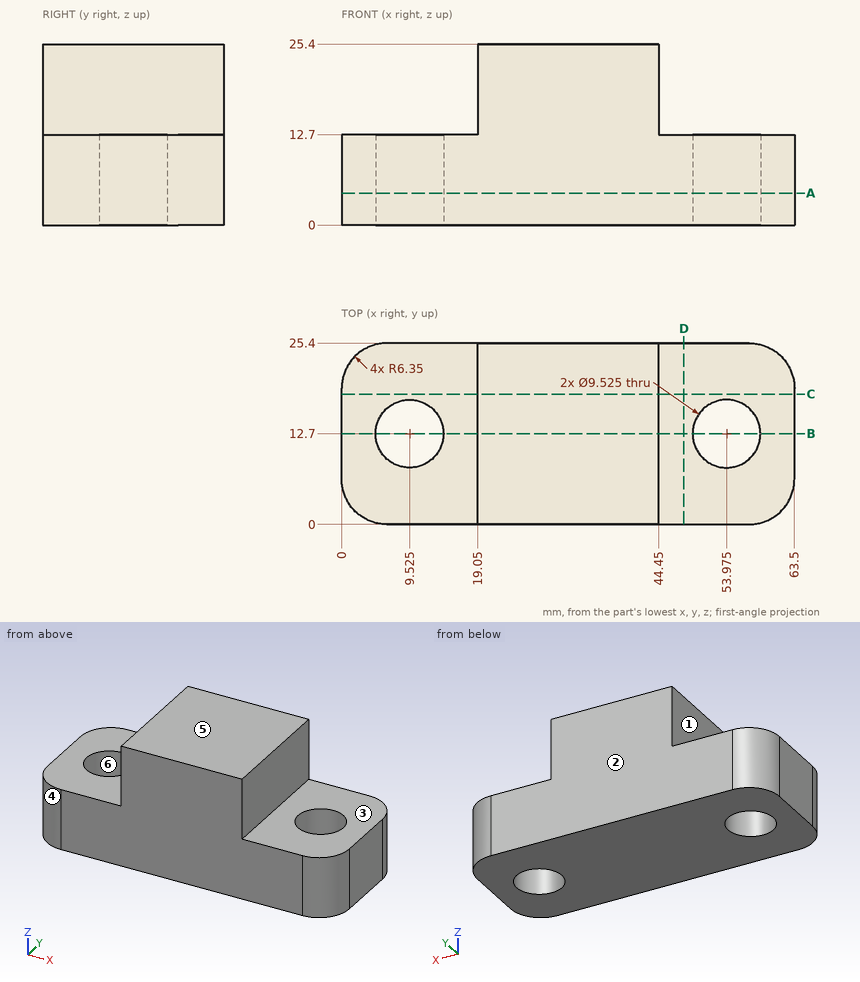
Could you check a few things on this drawing? It's one solid part, dimensions in mm from its lowest x, y, z. A direction names the side the tool comes from. Give positions to 0.01 mm unless a question says otherwise; leave off trailing zeros. Write each loop counter-clockwise with the first axis right and the second up, starting at its lowest first coordinate (ties: lowest second). Pieces come first, ordered by that corner, then holes. Notation, with made-up numbers: M -9.75,79.5 L 28.25,79.5 A29 ccw 28.25,118.5 Z; hole C -25,63 d8. An arc over 180 degrees is marked long. Put each result on its own line as item: value. Start each with the question number.
Item 1: If we section it at D-D, the plane x = 48: Write out the boundary of the cut face in (y, z).
Item 2: Will these pins go through, and if not, where does the flat tip stop? pin 1 (5 mm diameter, centred on x = 56.5, y = 11.5, fed in from -Z); pin 2 (7.5 mm diameter, centred on x = 53.975, y = 12.7, fed in from +Z); pin 3 (4 mm diameter, centred on y = 12, z = 19.5, fed in from +X); pin 4 (5.5 mm diameter, centred on x = 6, y = 14.5, fed in from +Z).
Item 3: Thinking about a two-plate mould opening in Y: for the marked faces 4, 5 and 6, which applies, +Y half, -Y half, draft (parallel to the pull), parting line (faces both ways), or undercut?
Item 4: If we section it at C-C, the plane y = 18.25: Write out the boundary of the cut face in (x, z), then the cut area to 3 significant figures.
Item 5: On a 3-axis mill with a long thin cutter (end or side, diameter ignored), from which of +Z, -Z, +X, -X, +Y, -Y can I reach the whole of each face in a straight line? I mean the marked faces 1, 2 and 3. Say none if no direction works.
Item 6: If we section it at A-A, the plane z = 4.5: Count the separate pieces of the cut face and the enclosed holes in it, then the cut area to 3 significant figures.
Item 7: I need wall thicknesses on L1, parallel to X at y = 15, z = 1.5; L2, parallel to X at y = 11, z = 8.75; L3, parallel to Z at x = 51.5, y = 22.75. Which ranges of each line are inside material? Lowest first, please. Write a range as from..to.
Item 8: If we section it at B-B, the plane y = 12.7: Write out the boundary of the cut face in (x, z).
Values:
1. outline: M 0,0 L 25.4,0 L 25.4,12.7 L 0,12.7 Z
2. pin 1: z = 0
2. pin 2: through
2. pin 3: x = 44.45
2. pin 4: z = 12.7
3. face 4: -Y half
3. face 5: draft
3. face 6: undercut
4. outline: M 0,0 L 63.5,0 L 63.5,12.7 L 44.45,12.7 L 44.45,25.4 L 19.05,25.4 L 19.05,12.7 L 0,12.7 Z
4. area: 1,130 mm²
5. face 1: +Z, -X, +Y, -Y
5. face 2: +Z, -Z, +X, -X, +Y
5. face 3: +Z, +X, +Y, -Y
6. separate pieces: 1
6. enclosed holes: 2
6. area: 1,440 mm²
7. L1: 0..5.35, 13.7..49.8, 58.15..63.5
7. L2: 0..5.08, 13.97..49.53, 58.42..63.5
7. L3: 0..12.7
8. outline: M 0,0 L 4.76,0 L 4.76,12.7 L 0,12.7 Z; M 14.29,0 L 49.21,0 L 49.21,12.7 L 44.45,12.7 L 44.45,25.4 L 19.05,25.4 L 19.05,12.7 L 14.29,12.7 Z; M 58.74,0 L 63.5,0 L 63.5,12.7 L 58.74,12.7 Z
